Source: CAD feature listing. Evaluate the final solid. Frame: model axes, mm. A direction names the side the tool comes from. Coordinates: 2 decimals unless noted, no trailing zeros. Order: outer loops, then holes, each group sorted by start corner. A loop starts at its lowest first (then second) coordinate and runs counter-clockwise, first axis right, second up.
```python
from build123d import *

# Parameters (mm, degrees)
F0_W        = 24
F0_H        = 26
F1_DEPTH    = 5
F2_T1_DEPTH = 5
F3_SIZE     = 1.5
F4_R        = 6
F5_SIZE     = 2
F6_R        = 0.75
F7_DEPTH    = 5
F8_DEPTH    = 2.5


# Not quite as in the source:
# - a fillet or chamfer that OpenCascade refuses, or shapes differently, is made with other operations: its cross-section is extruded or revolved along the edge and cut away or added


with BuildPart() as f1:
    # F0 (on Right) → F1 (new body)
    with BuildSketch(Plane.YZ):
        Rectangle(F0_W, F0_H)
        Polygon((22, 13), (12, 13), (12, -13), (12, -122), (22, -122), align=None)
    extrude(amount=F1_DEPTH)

    # F2: fillet of radius 25 on 1 edges, made by hand

    # F2_s2 → F2_t1 (join)
    with BuildSketch(Plane.YZ):
        with BuildLine():
            ThreePointArc((-12, -13), (5.0277563773, -20.6594839179), (12, -37.9799919936))
            Line((12, -37.9799919936), (12, -13))
            Line((12, -13), (-12, -13))
        make_face()
    extrude(amount=F2_T1_DEPTH)

    # F3
    f3_edges = [f1.edges().sort_by_distance(p)[0] for p in [
        (2.5, 12, -122),
        (2.5, 22, -122),
    ]]
    chamfer(f3_edges, length=F3_SIZE)

    # F4
    f4_edges = [f1.edges().sort_by_distance(p)[0] for p in [
        (2.5, -12, -13),
        (2.5, -12, 13),
        (2.5, 22, 13),
    ]]
    fillet(f4_edges, radius=F4_R)

    # F5
    f5_edges = [f1.edges().sort_by_distance(p)[0] for p in [
        (5, 22, -56.75),
        (0, 22, -56.75),
        (0, 6.572034, -22.425717),
        (0, -10.697288, -11.51368),
        (0, 12, -79.239996),
        (0, -12, -0.390327),
        (0, -10.242641, 11.242641),
        (0, 5, 13),
        (0, 20.242641, 11.242641),
        (5, 6.572034, -22.425717),
        (5, -10.697288, -11.51368),
        (5, 12, -79.239996),
        (5, -12, -0.390327),
        (5, -10.242641, 11.242641),
        (5, 5, 13),
        (5, 20.242641, 11.242641),
    ]]
    chamfer(f5_edges, length=F5_SIZE)

    # F6 (on face) → F7 (cut)
    with BuildSketch(Plane(origin=(0, 0, 0), x_dir=(0, -1, 0), z_dir=(-1, 0, 0))):
        with BuildLine():
            ThreePointArc((-2.8632404181, 3.5936789679), (-5.2698917444, 2.469041767), (-6.25, 0))
            ThreePointArc((-6.25, 0), (-5.2698917444, -2.469041767), (-2.8632404181, -3.5936789679))
            ThreePointArc((-2.8632404181, -3.5936789679), (-0.180958233, -2.6198917444), (0.95, 0))
            ThreePointArc((0.95, 0), (-0.180958233, 2.6198917444), (-2.8632404181, 3.5936789679))
        make_face()
        with BuildLine():
            ThreePointArc((-5.25, 0), (-2.65, 2.6), (-0.05, 0))
            ThreePointArc((-0.05, 0), (-2.65, -2.6), (-5.25, 0))
        make_face(mode=Mode.SUBTRACT)
        with BuildLine():
            ThreePointArc((-5.25, 0), (-2.65, -2.6), (-0.05, 0))
            ThreePointArc((-0.05, 0), (-2.65, 2.6), (-5.25, 0))
        make_face()
        with Locations((-17.65, 0)):
            Circle(F6_R)
        with BuildLine():
            Line((-16.4, 0), (-14.9, 0))
            ThreePointArc((-14.9, 0), (-15.65, 0.75), (-16.4, 0))
        make_face()
        with BuildLine():
            ThreePointArc((-16.4, 0), (-15.65, -0.75), (-14.9, 0))
            Line((-14.9, 0), (-16.4, 0))
        make_face()
        with BuildLine():
            ThreePointArc((-10.9, 0), (-11.65, 0.75), (-12.4, 0))
            Line((-12.4, 0), (-10.9, 0))
        make_face()
        with BuildLine():
            Line((-10.9, 0), (-12.4, 0))
            ThreePointArc((-12.4, 0), (-11.65, -0.75), (-10.9, 0))
        make_face()
        with BuildLine():
            ThreePointArc((-10.4, 0), (-9.65, -0.75), (-8.9, 0))
            Line((-8.9, 0), (-10.4, 0))
        make_face()
        with BuildLine():
            Line((-10.4, 0), (-8.9, 0))
            ThreePointArc((-8.9, 0), (-9.65, 0.75), (-10.4, 0))
        make_face()
        with BuildLine():
            Line((-8.4, 0), (-6.9, 0))
            ThreePointArc((-6.9, 0), (-7.65, 0.75), (-8.4, 0))
        make_face()
        with BuildLine():
            ThreePointArc((-8.4, 0), (-7.65, -0.75), (-6.9, 0))
            Line((-6.9, 0), (-8.4, 0))
        make_face()
        with BuildLine():
            ThreePointArc((-12.9, 0), (-13.4380659424, 0.719433079), (-14.2802238806, 0.406592991))
            ThreePointArc((-14.2802238806, 0.406592991), (-14.2575663793, 0.2038573909), (-14.25, 0))
            Line((-14.25, 0), (-12.9, 0))
        make_face()
        with BuildLine():
            ThreePointArc((-14.25, 0), (-14.2575663793, -0.2038573909), (-14.2802238806, -0.406592991))
            ThreePointArc((-14.2802238806, -0.406592991), (-13.4380659424, -0.719433079), (-12.9, 0))
            Line((-12.9, 0), (-14.25, 0))
        make_face()
        with BuildLine():
            ThreePointArc((-14.4, 0), (-14.369433079, -0.2119340576), (-14.2802238806, -0.406592991))
            ThreePointArc((-14.2802238806, -0.406592991), (-14.2575663793, -0.2038573909), (-14.25, 0))
            Line((-14.25, 0), (-14.4, 0))
        make_face()
        with BuildLine():
            ThreePointArc((-14.25, 0), (-14.2575663793, 0.2038573909), (-14.2802238806, 0.406592991))
            ThreePointArc((-14.2802238806, 0.406592991), (-14.369433079, 0.2119340576), (-14.4, 0))
            Line((-14.4, 0), (-14.25, 0))
        make_face()
    extrude(amount=-F7_DEPTH, mode=Mode.SUBTRACT)

    # F6 (on face) → F8 (cut)
    with BuildSketch(Plane(origin=(0, 0, 0), x_dir=(0, -1, 0), z_dir=(-1, 0, 0))):
        with BuildLine():
            ThreePointArc((-2.8632404181, -3.5936789679), (-5.2698917444, -2.469041767), (-6.25, 0))
            Line((-6.25, 0), (-6.9, 0))
            ThreePointArc((-6.9, 0), (-7.65, -0.75), (-8.4, 0))
            Line((-8.4, 0), (-8.9, 0))
            ThreePointArc((-8.9, 0), (-9.65, -0.75), (-10.4, 0))
            Line((-10.4, 0), (-10.9, 0))
            ThreePointArc((-10.9, 0), (-11.65, -0.75), (-12.4, 0))
            Line((-12.4, 0), (-12.9, 0))
            ThreePointArc((-12.9, 0), (-13.4380659424, -0.719433079), (-14.2802238806, -0.406592991))
            ThreePointArc((-14.2802238806, -0.406592991), (-15.2674725396, -2.1356143376), (-17.1628919861, -2.7451714338))
            Line((-17.1628919861, -2.7451714338), (-2.8632404181, -3.5936789679))
        make_face()
        with BuildLine():
            ThreePointArc((-14.2802238806, 0.406592991), (-15.2674725396, 2.1356143376), (-17.1628919861, 2.7451714338))
            ThreePointArc((-17.1628919861, 2.7451714338), (-19.75, 0), (-17.1628919861, -2.7451714338))
            ThreePointArc((-17.1628919861, -2.7451714338), (-15.2674725396, -2.1356143376), (-14.2802238806, -0.406592991))
            ThreePointArc((-14.2802238806, -0.406592991), (-14.369433079, -0.2119340576), (-14.4, 0))
            ThreePointArc((-14.4, 0), (-14.369433079, 0.2119340576), (-14.2802238806, 0.406592991))
        make_face()
        with Locations((-17.65, 0)):
            Circle(F6_R, mode=Mode.SUBTRACT)
        with BuildLine():
            ThreePointArc((-16.4, 0), (-15.65, 0.75), (-14.9, 0))
            ThreePointArc((-14.9, 0), (-15.65, -0.75), (-16.4, 0))
        make_face(mode=Mode.SUBTRACT)
        with BuildLine():
            Line((-6.9, 0), (-6.25, 0))
            ThreePointArc((-6.25, 0), (-5.2698917444, 2.469041767), (-2.8632404181, 3.5936789679))
            Line((-2.8632404181, 3.5936789679), (-17.1628919861, 2.7451714338))
            ThreePointArc((-17.1628919861, 2.7451714338), (-15.2674725396, 2.1356143376), (-14.2802238806, 0.406592991))
            ThreePointArc((-14.2802238806, 0.406592991), (-13.4380659424, 0.719433079), (-12.9, 0))
            Line((-12.9, 0), (-12.4, 0))
            ThreePointArc((-12.4, 0), (-11.65, 0.75), (-10.9, 0))
            Line((-10.9, 0), (-10.4, 0))
            ThreePointArc((-10.4, 0), (-9.65, 0.75), (-8.9, 0))
            Line((-8.9, 0), (-8.4, 0))
            ThreePointArc((-8.4, 0), (-7.65, 0.75), (-6.9, 0))
        make_face()
    extrude(amount=-F8_DEPTH, mode=Mode.SUBTRACT)


solid = f1.part
```
Q1. Set-up query: faces 1 (the flat face through (1.232, 10.113, -3.163)), 2 (the conical face through (0.792, -9.351, 10.425)). Return all of +Z, -Z, +X, -X, +Y, -Y with unobstructed straight access to the full face (end or side cutting, diameter ignored); none if empty.
Solutions:
face 1: -X
face 2: +Z, -X, -Y
Q2. Section query A-A on z = -46. Output: boundary loops of the cut face in (x, y).
Solutions:
outline: (0, 14) - (2, 12) - (3, 12) - (5, 14) - (5, 20) - (3, 22) - (2, 22) - (0, 20) - close
Q3. Material intervals for line 1 along Y through (x, z) = (3.45, -2); line 2 along Z through (x, y) = (4.25, 15); line 3 along Z through (x, y) = (3.15, 7.65), sorted ascending.
Solutions:
line 1: y = -11.55 to -0.34, 5.64 to 21.55
line 2: z = -122 to -0.37, 0.37 to 11.75
line 3: z = -23.62 to -0.75, 0.75 to 12.85
Q4. Pull-direction query (Z, two-part tool) for faces 3 (the flat face through (0, 11, -25)), 4 (the cylindrical face through (2.493, 6.425, -22.242)), 5 (the flat face through (1.232, 9.913, 3.175)), 6 (the cylindrical face through (1.23, 19.75, 0.06)); classes: pulls with the +Z half, pulls with the -Z half, needs draft (parallel to the pull), parting line crosses it, or undercut.
Solutions:
face 3: needs draft
face 4: pulls with the -Z half
face 5: undercut
face 6: undercut
Q5. Pin query (flat end, axial travel): P1, Ø1.4, axis at y = 11.65, z = 0, coming from the -X side; P2, Ø2, axis at y = 9.65, z = 0, coming from the -X side; P3, Ø0.5, axis at x = 2.5, z = -71.5, coming from the -Y side. Return the tip coordinate at first contact, or that it passes through.
Solutions:
P1: passes through
P2: stops at x = 2.5
P3: stops at y = 12
